Work out the finished part from the listing and answer in its coordinate system (mm). Face numbers are marked on the shaded views. A direction names the side the tool comes from. Coordinates: 2 decimals unless noted, no trailing zeros. Write each loop counter-clockwise with the first axis right and the second up, starting at its lowest first coordinate (ties: lowest second). Pieces come first, ordered by that corner, then holes. Notation, with made-up numbers: (56.25, -18.75) - (107.25, -18.75) arc R25 ccw to (107.25, -2.75) - close; hole circle Ø10 at (-33.75, 41.5). An arc over 180 degrees is marked (long way). Use a Markdown table: item, result. Add a question column.
(1) Find the intervals of material crossed by line 1 (X direction, y = -0.25, z = 2.75); line 2 (X direction, y = 2.5, z = -6.25); line 3 (Y direction, x = 0, z = 2), in increasing order. Write a range as from..to.
(2) A tool of negligible diameter and unlimited length cuts with its end or side. For the marked faces 1 and 2, from which of +Z, -Z, +X, -X, +Y, -Y can it reach the whole face along a straight path? Write none if from no direction.
(3) The part is cut by section A-A, the plane x = 20. Give the vertices of the cut face in (y, z).
(4) Given pin 1 Ø1.8 at (y, z) = (7, -1.5) entering from +X; pin 2 Ø6 at (x, z) = (3, 3.5) entering from -Y; pin 3 Ø1.8 at (y, z) = (6.5, -0.5) entering from -X, each flat-ended and moving along its own axis, determine where each tip first touches the part or whether it passes through.
(5) For a pull along X with two mould halves and no side action, classify the marked faces 3, 4 and 5 as released by +X, released by -X, zero draft, split by the parting line, or undercut.
(6) The part is cut by section C-C, the plane z = -4.5. Give the vertices of the cut face in (x, y).
(7) The part is cut by section B-B, the plane y = 6.25. Give the vertices of the cut face in (x, z).
(8) The part is cut by section D-D, the plane x = 0. Give the vertices of the cut face in (y, z).
from build123d import *

# Parameters (mm, degrees)
BOSS_EXTRUDE1_DEPTH = 12.5
CUT_EXTRUDE1_DEPTH  = 5.628
FILLET5_R           = 2
CHAMFER9_SIZE       = 2
SKETCH4_R           = 2.64775
BOSS_EXTRUDE2_DEPTH = 4.4055


with BuildPart() as part:
    # Sketch1 → Boss-Extrude1 (new body, symmetric)
    with BuildSketch(Plane.XY):
        with BuildLine():
            Line((-25, 0), (-15, 0))
            ThreePointArc((-15, 0), (0, 15), (15, 0))
            Line((15, 0), (25, 0))
            ThreePointArc((25, 0), (0, 25), (-25, 0))
        make_face()
    extrude(amount=BOSS_EXTRUDE1_DEPTH, both=True)

    # Sketch3 → Cut-Extrude1 (cut, symmetric)
    with BuildSketch(Plane(origin=(0, 0, 0), x_dir=(-1, 0, 0), z_dir=(0, 0, -1))):
        with BuildLine():
            Line((15, 0), (15.5936, 0))
            Line((15.5936, 0), (15.5936, 4.536))
            Line((15.5936, 4.536), (16.6576, 5.712))
            Line((16.6576, 5.712), (16.6576, 8.008))
            Line((16.6576, 8.008), (12.683530108, 8.008))
            ThreePointArc((12.683530108, 8.008), (14.409249662, 4.16815597), (15, 0))
        make_face()
    cut_extrude1 = extrude(amount=CUT_EXTRUDE1_DEPTH, both=True, mode=Mode.SUBTRACT)

    # Mirror3: Cut-Extrude1 across plane
    add(cut_extrude1.mirror(Plane(origin=(0, 0, 0), x_dir=(0, 0, 1), z_dir=(1, 0, 0))), mode=Mode.SUBTRACT)

    # Fillet5
    fillet5_edges = [part.edges().sort_by_distance(p)[0] for p in [
        (-15.5936, 4.536, 0),
        (15.5936, 4.536, 0),
    ]]
    fillet(fillet5_edges, radius=FILLET5_R)

    # Chamfer9
    chamfer9_edges = [part.edges().sort_by_distance(p)[0] for p in [
        (-15.5936, 0, 0),
        (15.5936, 0, 0),
    ]]
    chamfer(chamfer9_edges, length=CHAMFER9_SIZE)

    # Sketch4 → Boss-Extrude2 (add)
    with BuildSketch(Plane.XZ):
        with Locations((-20, 4.5)):
            Circle(SKETCH4_R)
        with Locations((-20, -4.5)):
            Circle(SKETCH4_R)
    boss_extrude2 = extrude(amount=BOSS_EXTRUDE2_DEPTH)

    # Mirror4: Boss-Extrude2 across plane
    add(boss_extrude2.mirror(Plane(origin=(0, 0, 0), x_dir=(0, 0, 1), z_dir=(1, 0, 0))))


solid = part.part
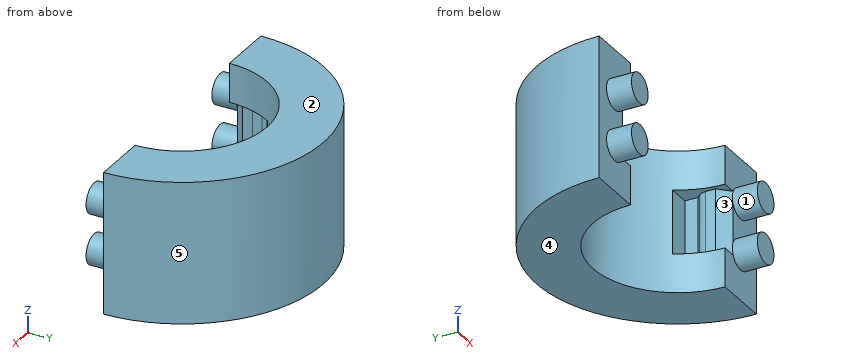
Model answer:
| question | item | result |
|---|---|---|
| 1 | line 1 | -21.99..-18.01, 18.01..21.99 |
| 1 | line 2 | -24.87..-14.79, 14.79..24.87 |
| 1 | line 3 | 15..25 |
| 2 | face 1 | -Y |
| 2 | face 2 | +Z, +X, -X, +Y, -Y |
| 3 | outline | (-4.41, -7.15) - (0, -7.15) - (0, -12.5) - (15, -12.5) - (15, 12.5) - (0, 12.5) - (0, 7.15) - (-4.41, 7.15) - (-4.41, 1.85) - (0, 1.85) - (0, -1.85) - (-4.41, -1.85) - close |
| 4 | pin 1 | x = 24.24 |
| 4 | pin 2 | y = 13.75 |
| 4 | pin 3 | x = -24.36 |
| 5 | face 3 | undercut |
| 5 | face 4 | zero draft |
| 5 | face 5 | split by the parting line |
| 6 | outline | (-25, 0) - (-22.65, 0) - (-22.65, -4.41) - (-17.35, -4.41) - (-17.35, 0) - (-17.59, 0) - (-15.59, 2) - (-15.59, 3.77) arc R2 ccw to (-16.11, 5.11) - (-16.66, 5.71) - (-16.66, 8.01) - (-12.68, 8.01) arc R15 cw to (12.68, 8.01) - (16.66, 8.01) - (16.66, 5.71) - (16.11, 5.11) arc R2 ccw to (15.59, 3.77) - (15.59, 2) - (17.59, 0) - (17.35, 0) - (17.35, -4.41) - (22.65, -4.41) - (22.65, 0) - (25, 0) arc R25 ccw to start |
| 7 | outline | (-24.21, -12.5) - (-13.64, -12.5) - (-13.64, -5.63) - (-16.66, -5.63) - (-16.66, 5.63) - (-13.64, 5.63) - (-13.64, 12.5) - (-24.21, 12.5) - close; (13.64, -12.5) - (24.21, -12.5) - (24.21, 12.5) - (13.64, 12.5) - (13.64, 5.63) - (16.66, 5.63) - (16.66, -5.63) - (13.64, -5.63) - close |
| 8 | outline | (15, -12.5) - (25, -12.5) - (25, 12.5) - (15, 12.5) - close |
